from build123d import *

# Parameters (mm, degrees)
SKETCH_1_W      = 93.979995727
SKETCH_1_H      = 24.130004883
SKETCH_1_R      = 1.25000004
SKETCH_1_R_2    = 0.3999992
SKETCH_1_R_3    = 0.5499989
SKETCH_1_R_4    = 0.4499991
SKETCH_1_R_5    = 0.3499993
EXTRUDE_1_DEPTH = 1.5


with BuildPart() as part:
    # Эскиз1 → Бобышка-Вытянуть1 (new body)
    with BuildSketch(Plane(origin=(0, 0, -0.34544), x_dir=(-1, 0, 0), z_dir=(0, 0, -1))):
        with Locations((-119.379997253, 83.819999695)):
            Rectangle(SKETCH_1_W, SKETCH_1_H)
        with Locations(Location((-163.195, 92.71, 0), (0, 0, 180))):
            Circle(SKETCH_1_R, mode=Mode.SUBTRACT)
        with Locations(Location((-154.6499828, 88.81999, 0), (0, 0, 180))):
            Circle(SKETCH_1_R_2, mode=Mode.SUBTRACT)
        with Locations(Location((-162.56, 86.36, 0), (0, 0, 180))):
            Circle(SKETCH_1_R_3, mode=Mode.SUBTRACT)
        with Locations(Location((-154.6499828, 86.3200204, 0), (0, 0, 180))):
            Circle(SKETCH_1_R_2, mode=Mode.SUBTRACT)
        with Locations(Location((-154.6499828, 83.82, 0), (0, 0, 180))):
            Circle(SKETCH_1_R_2, mode=Mode.SUBTRACT)
        with Locations(Location((-104.775, 85.05001786, 0), (0, 0, 180))):
            Circle(SKETCH_1_R_2, mode=Mode.SUBTRACT)
        with Locations(Location((-126.907544, 83.185, 0), (0, 0, 180))):
            Circle(SKETCH_1_R_2, mode=Mode.SUBTRACT)
        with Locations(Location((-104.77500254, 82.55, 0), (0, 0, 180))):
            Circle(SKETCH_1_R_2, mode=Mode.SUBTRACT)
        with Locations(Location((-162.56, 81.28, 0), (0, 0, 180))):
            Circle(SKETCH_1_R_3, mode=Mode.SUBTRACT)
        with Locations(Location((-154.6499828, 81.3199796, 0), (0, 0, 180))):
            Circle(SKETCH_1_R_2, mode=Mode.SUBTRACT)
        with Locations(Location((-163.195, 74.93, 0), (0, 0, 180))):
            Circle(SKETCH_1_R, mode=Mode.SUBTRACT)
        with Locations(Location((-154.6499828, 78.82001, 0), (0, 0, 180))):
            Circle(SKETCH_1_R_2, mode=Mode.SUBTRACT)
        with Locations(Location((-126.907544, 80.645, 0), (0, 0, 180))):
            Circle(SKETCH_1_R_2, mode=Mode.SUBTRACT)
        with Locations(Location((-101.329998, 79.7799776, 0), (0, 0, 180))):
            Circle(SKETCH_1_R_4, mode=Mode.SUBTRACT)
        with Locations(Location((-126.907544, 75.565, 0), (0, 0, 180))):
            Circle(SKETCH_1_R_2, mode=Mode.SUBTRACT)
        with Locations(Location((-126.907544, 78.105, 0), (0, 0, 180))):
            Circle(SKETCH_1_R_2, mode=Mode.SUBTRACT)
        with Locations(Location((-85.725, 87.63, 0), (0, 0, 180))):
            Circle(SKETCH_1_R_2, mode=Mode.SUBTRACT)
        with Locations(Location((-83.185, 87.63, 0), (0, 0, 180))):
            Circle(SKETCH_1_R_2, mode=Mode.SUBTRACT)
        with Locations(Location((-85.725, 82.55, 0), (0, 0, 180))):
            Circle(SKETCH_1_R_2, mode=Mode.SUBTRACT)
        with Locations(Location((-85.725, 85.09, 0), (0, 0, 180))):
            Circle(SKETCH_1_R_2, mode=Mode.SUBTRACT)
        with Locations(Location((-80.01, 87.63, 0), (0, 0, 180))):
            Circle(SKETCH_1_R_5, mode=Mode.SUBTRACT)
        with Locations(Location((-75.565, 92.71, 0), (0, 0, 180))):
            Circle(SKETCH_1_R, mode=Mode.SUBTRACT)
        with Locations(Location((-83.185, 85.09, 0), (0, 0, 180))):
            Circle(SKETCH_1_R_2, mode=Mode.SUBTRACT)
        with Locations(Location((-76.2, 86.36, 0), (0, 0, 180))):
            Circle(SKETCH_1_R_3, mode=Mode.SUBTRACT)
        with Locations(Location((-85.725, 80.01, 0), (0, 0, 180))):
            Circle(SKETCH_1_R_2, mode=Mode.SUBTRACT)
        with Locations(Location((-83.185, 82.55, 0), (0, 0, 180))):
            Circle(SKETCH_1_R_2, mode=Mode.SUBTRACT)
        with Locations(Location((-93.330014, 79.7799776, 0), (0, 0, 180))):
            Circle(SKETCH_1_R_4, mode=Mode.SUBTRACT)
        with Locations(Location((-83.185, 80.01, 0), (0, 0, 180))):
            Circle(SKETCH_1_R_2, mode=Mode.SUBTRACT)
        with Locations(Location((-80.01, 80.0300152, 0), (0, 0, 180))):
            Circle(SKETCH_1_R_5, mode=Mode.SUBTRACT)
        with Locations(Location((-76.2, 81.28, 0), (0, 0, 180))):
            Circle(SKETCH_1_R_3, mode=Mode.SUBTRACT)
        with Locations(Location((-75.565, 74.93, 0), (0, 0, 180))):
            Circle(SKETCH_1_R, mode=Mode.SUBTRACT)
    extrude(amount=-EXTRUDE_1_DEPTH)


solid = part.part
Can you work these out from the model? Positions are in its coordinate system, mm. Give positions to 0.01 mm unless a question says otherwise; leave off trailing zeros. One line per question, with ' | ' between items.
Item 1: Please list where these lines run through material, in increasing order: L1, parallel to X at y = 74.75, z = 0.7; L2, parallel to X at y = 86.36, z = 0.05; L3, parallel to X at y = 92.71, z = 0.85 (3 decimals).
Answer block:
L1: x = 72.39 to 74.33, 76.8 to 161.96, 164.43 to 166.37 | L2: x = 72.39 to 75.65, 76.75 to 154.25, 155.05 to 162.01, 163.11 to 166.37 | L3: x = 72.39 to 74.315, 76.815 to 161.945, 164.445 to 166.37
Item 2: I'm going to push a flat-ended pin straight in: pin 1 Ø2 at (x, y) = (163.195, 74.93) entering from +Z. Where does the tip first touch, or does it pass through?
Answer block:
pin 1: passes through
Item 3: Suppose I cut it at A-A, the plane z = 0.8. Give the number of separate pieces and of enclosed holes in the cut face, then the cut area to 3 significant figures.
Answer block:
separate pieces: 1 | enclosed holes: 31 | area: 2,230 mm2
Item 4: We'd pull the mould along X, two halves only. Please class faces 1 (the face through (72.39, 84, 0)), 2 (the face through (76.14, 93.82, 0.39)), 3 (the face through (162.203, 93.471, 0.394)), 4 (the face through (120, 84, -0.345)): released by +X, released by -X, zero draft, split by the parting line, or undercut.
Answer block:
face 1: released by -X | face 2: undercut | face 3: undercut | face 4: zero draft
